The figure shows three views and two pictorial views of one solid part (mm, origin at its lowest corner). Answer the questions. A direction names the side the tool comes from. Coordinates: 2 decimals unless noted, no trailing zeros. Loops run counter-clockwise (first coordinate to the right, second up) from the corner with the lowest first, then second, coordinate; pieces in that order, holes last. Notation, with made-up numbers: (74, 36.25) -> (118, 36.25) arc R29 cw to (118, 59.25) -> close; hole circle Ø11 at (71.25, 81.5). An arc over 180 degrees is marked (long way). Answer as a JSON object with one key per item and string values. Group by question number.
1) Consider probe 1 along X at (y, z) = (0.65, 13); probe 2 along Z at (x, y) = (15.5, 0.5); probe 3 along X at (y, z) = (2.9, 10.25). Determine where each line is inside the solid, lowest interval first. Write a range as [from, to].
2) Section C-C, the plane y = 2.7 is taken. Give the vertices of the cut face in (x, z).
3) Determine the mould class of the marked faces 1, 2, 3 and 4 for opening direction X: released by +X, released by -X, zero draft, split by the parting line, or undercut.
4) Section B-B, the plane x = 26.5 is taken. Give the vertices of the cut face in (y, z).
5) Flat-ended cylindrical pins translate along their axes: P1, Ø5.5, axis at x = 8.5, z = 9, coming from the +Y side; P2, Ø0.6, axis at x = 35.5, y = 1, coming from the -Z side. Find the tip coordinate at first contact, or state that the pin passes through.
6) Section D-D, the plane x = 10 is taken. Give the vertices of the cut face in (y, z).
7) Section A-A, the plane z = 14 is taken. Give the vertices of the cut face in (x, y).
8) Which of the six approach directions +Z, -Z, +X, -X, +Y, -Y give full straight-line access (tool end or side, diameter ignored) to the marked faces 5 and 6?
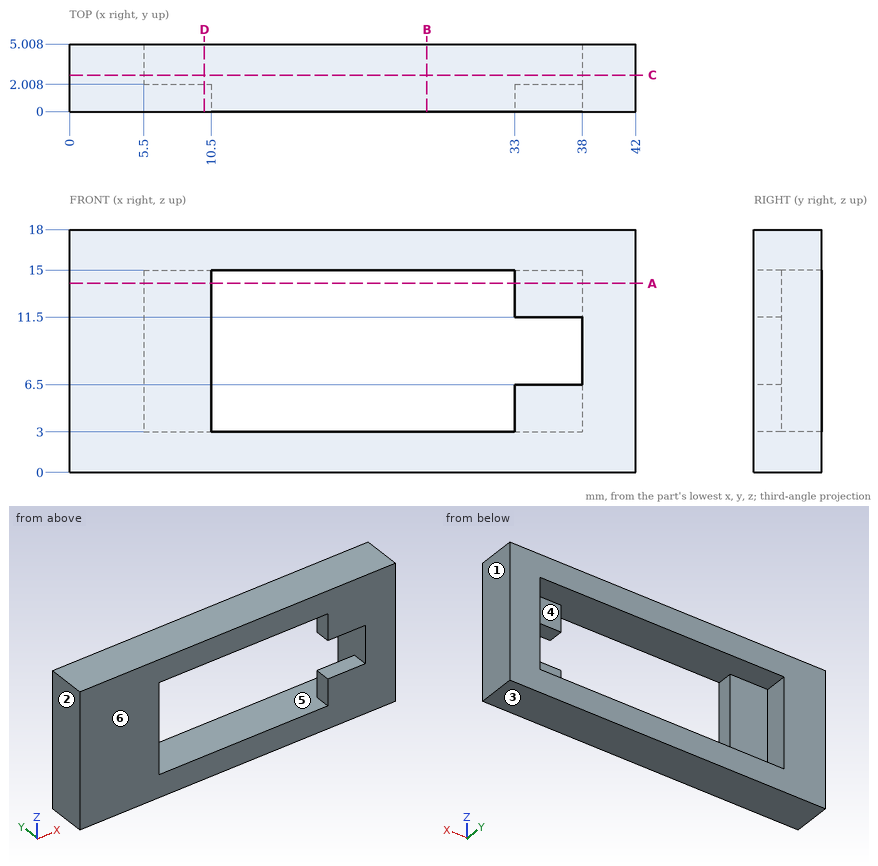
Determined:
{
 "1": {"probe 1": "[0, 10.5], [33, 42]", "probe 2": "[0, 3], [15, 18]", "probe 3": "[0, 5.5], [38, 42]"},
 "2": {"outline": "(0, 0) -> (42, 0) -> (42, 18) -> (0, 18) -> close; hole (5.5, 3) -> (38, 3) -> (38, 15) -> (5.5, 15) -> close"},
 "3": {"face 1": "released by +X", "face 2": "released by -X", "face 3": "zero draft", "face 4": "undercut"},
 "4": {"outline": "(0, 0) -> (5.01, 0) -> (5.01, 3) -> (0, 3) -> close; (0, 15) -> (5.01, 15) -> (5.01, 18) -> (0, 18) -> close"},
 "5": {"P1": "y = 2.01", "P2": "z = 0"},
 "6": {"outline": "(0, 0) -> (5.01, 0) -> (5.01, 3) -> (2.01, 3) -> (2.01, 15) -> (5.01, 15) -> (5.01, 18) -> (0, 18) -> close"},
 "7": {"outline": "(0, 0) -> (10.5, 0) -> (10.5, 2.01) -> (5.5, 2.01) -> (5.5, 5.01) -> (0, 5.01) -> close; (33, 0) -> (42, 0) -> (42, 5.01) -> (38, 5.01) -> (38, 2.01) -> (33, 2.01) -> close"},
 "8": {"face 5": "+Y", "face 6": "+Z, -Z, +X, -X, -Y"}
}
